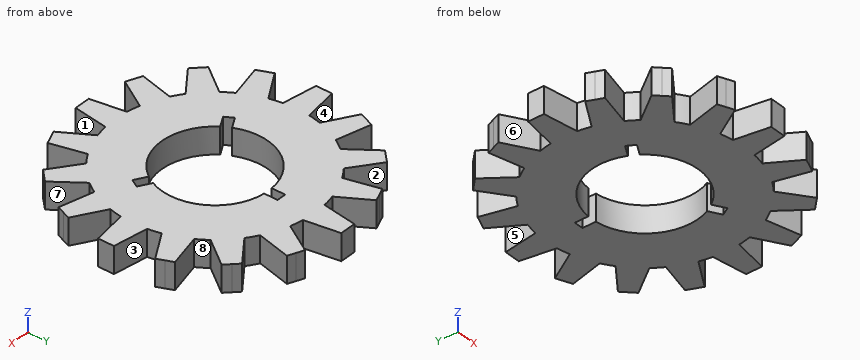
from build123d import *

# Parameters (mm, degrees)
F1_DEPTH = 2.54


with BuildPart() as f1:
    # F0 (on Top) → F1 (new body)
    with BuildSketch(Plane.XY):
        with BuildLine():
            Line((-9.5190714883, 8.4414407538), (-7.564357968, 5.788446556))
            ThreePointArc((-7.564357968, 5.788446556), (-7.9197480572, 5.2918064695), (-8.242581769, 4.7734129071))
            Line((-8.242581769, 4.7734129071), (-11.4416652874, 5.5640757948))
            Line((-11.4416652874, 5.5640757948), (-11.7332700629, 4.860079591))
            Line((-11.7332700629, 4.860079591), (-12.0248748384, 4.1560833873))
            Line((-12.0248748384, 4.1560833873), (-9.2036980994, 2.4530728273))
            ThreePointArc((-9.2036980994, 2.4530728273), (-9.3419797958, 1.8582353172), (-9.4418586268, 1.2557590022))
            Line((-9.4418586268, 1.2557590022), (-12.7, 0.762))
            Line((-12.7, 0.762), (-12.7, 0))
            Line((-12.7, 0), (-12.7, -0.762))
            Line((-12.7, -0.762), (-9.4418586268, -1.2557590022))
            ThreePointArc((-9.4418586268, -1.2557590022), (-9.3419797958, -1.8582353172), (-9.2036980994, -2.4530728273))
            Line((-9.2036980994, -2.4530728273), (-12.0248748384, -4.1560833873))
            Line((-12.0248748384, -4.1560833873), (-11.7332700629, -4.860079591))
            Line((-11.7332700629, -4.860079591), (-11.4416652874, -5.5640757948))
            Line((-11.4416652874, -5.5640757948), (-8.242581769, -4.7734129071))
            ThreePointArc((-8.242581769, -4.7734129071), (-7.9197480572, -5.2918064695), (-7.564357968, -5.788446556))
            Line((-7.564357968, -5.788446556), (-9.5190714883, -8.4414407538))
            Line((-9.5190714883, -8.4414407538), (-8.9802561211, -8.9802561211))
            Line((-8.9802561211, -8.9802561211), (-8.4414407538, -9.5190714883))
            Line((-8.4414407538, -9.5190714883), (-5.788446556, -7.564357968))
            ThreePointArc((-5.788446556, -7.564357968), (-5.2918064695, -7.9197480572), (-4.7734129071, -8.242581769))
            Line((-4.7734129071, -8.242581769), (-5.5640757948, -11.4416652874))
            Line((-5.5640757948, -11.4416652874), (-4.860079591, -11.7332700629))
            Line((-4.860079591, -11.7332700629), (-4.1560833873, -12.0248748384))
            Line((-4.1560833873, -12.0248748384), (-2.4530728273, -9.2036980994))
            ThreePointArc((-2.4530728273, -9.2036980994), (-1.8582353172, -9.3419797958), (-1.2557590022, -9.4418586268))
            Line((-1.2557590022, -9.4418586268), (-0.762, -12.7))
            Line((-0.762, -12.7), (0, -12.7))
            Line((0, -12.7), (0.762, -12.7))
            Line((0.762, -12.7), (1.2557590022, -9.4418586268))
            ThreePointArc((1.2557590022, -9.4418586268), (1.8582353172, -9.3419797958), (2.4530728273, -9.2036980994))
            Line((2.4530728273, -9.2036980994), (4.1560833873, -12.0248748384))
            Line((4.1560833873, -12.0248748384), (4.860079591, -11.7332700629))
            Line((4.860079591, -11.7332700629), (5.5640757948, -11.4416652874))
            Line((5.5640757948, -11.4416652874), (4.7734129071, -8.242581769))
            ThreePointArc((4.7734129071, -8.242581769), (5.2918064695, -7.9197480572), (5.788446556, -7.564357968))
            Line((5.788446556, -7.564357968), (8.4414407538, -9.5190714883))
            Line((8.4414407538, -9.5190714883), (8.9802561211, -8.9802561211))
            Line((8.9802561211, -8.9802561211), (9.5190714883, -8.4414407538))
            Line((9.5190714883, -8.4414407538), (7.564357968, -5.788446556))
            ThreePointArc((7.564357968, -5.788446556), (7.9197480572, -5.2918064695), (8.242581769, -4.7734129071))
            Line((8.242581769, -4.7734129071), (11.4416652874, -5.5640757948))
            Line((11.4416652874, -5.5640757948), (11.7332700629, -4.860079591))
            Line((11.7332700629, -4.860079591), (12.0248748384, -4.1560833873))
            Line((12.0248748384, -4.1560833873), (9.2036980994, -2.4530728273))
            ThreePointArc((9.2036980994, -2.4530728273), (9.3419797958, -1.8582353172), (9.4418586268, -1.2557590022))
            Line((9.4418586268, -1.2557590022), (12.7, -0.762))
            Line((12.7, -0.762), (12.7, 0))
            Line((12.7, 0), (12.7, 0.762))
            Line((12.7, 0.762), (9.4418586268, 1.2557590022))
            ThreePointArc((9.4418586268, 1.2557590022), (9.3419797958, 1.8582353172), (9.2036980994, 2.4530728273))
            Line((9.2036980994, 2.4530728273), (12.0248748384, 4.1560833873))
            Line((12.0248748384, 4.1560833873), (11.7332700629, 4.860079591))
            Line((11.7332700629, 4.860079591), (11.4416652874, 5.5640757948))
            Line((11.4416652874, 5.5640757948), (8.242581769, 4.7734129071))
            ThreePointArc((8.242581769, 4.7734129071), (7.9197480572, 5.2918064695), (7.564357968, 5.788446556))
            Line((7.564357968, 5.788446556), (9.5190714883, 8.4414407538))
            Line((9.5190714883, 8.4414407538), (8.9802561211, 8.9802561211))
            Line((8.9802561211, 8.9802561211), (8.4414407538, 9.5190714883))
            Line((8.4414407538, 9.5190714883), (5.788446556, 7.564357968))
            ThreePointArc((5.788446556, 7.564357968), (5.2918064695, 7.9197480572), (4.7734129071, 8.242581769))
            Line((4.7734129071, 8.242581769), (5.5640757948, 11.4416652874))
            Line((5.5640757948, 11.4416652874), (4.860079591, 11.7332700629))
            Line((4.860079591, 11.7332700629), (4.1560833873, 12.0248748384))
            Line((4.1560833873, 12.0248748384), (2.4530728273, 9.2036980994))
            ThreePointArc((2.4530728273, 9.2036980994), (1.8582353172, 9.3419797958), (1.2557590022, 9.4418586268))
            Line((1.2557590022, 9.4418586268), (0.762, 12.7))
            Line((0.762, 12.7), (0, 12.7))
            Line((0, 12.7), (-0.762, 12.7))
            Line((-0.762, 12.7), (-1.2557590022, 9.4418586268))
            ThreePointArc((-1.2557590022, 9.4418586268), (-1.8582353172, 9.3419797958), (-2.4530728273, 9.2036980994))
            Line((-2.4530728273, 9.2036980994), (-4.1560833873, 12.0248748384))
            Line((-4.1560833873, 12.0248748384), (-4.860079591, 11.7332700629))
            Line((-4.860079591, 11.7332700629), (-5.5640757948, 11.4416652874))
            Line((-5.5640757948, 11.4416652874), (-4.7734129071, 8.242581769))
            ThreePointArc((-4.7734129071, 8.242581769), (-5.2918064695, 7.9197480572), (-5.788446556, 7.564357968))
            Line((-5.788446556, 7.564357968), (-8.4414407538, 9.5190714883))
            Line((-8.4414407538, 9.5190714883), (-8.9802561211, 8.9802561211))
            Line((-8.9802561211, 8.9802561211), (-9.5190714883, 8.4414407538))
        make_face()
        with BuildLine():
            ThreePointArc((-4.6047852038, -2.1453095877), (-4.3994090512, 2.54), (-0.4445, 5.0605157593))
            Line((-0.4445, 5.0605157593), (-0.4445, 6.35))
            Line((-0.4445, 6.35), (0, 6.35))
            Line((0, 6.35), (0.4445, 6.35))
            Line((0.4445, 6.35), (0.4445, 5.0605157593))
            ThreePointArc((0.4445, 5.0605157593), (4.3994090512, 2.54), (4.6047852038, -2.1453095877))
            Line((4.6047852038, -2.1453095877), (5.721511314, -2.790051708))
            Line((5.721511314, -2.790051708), (5.277011314, -3.559948292))
            Line((5.277011314, -3.559948292), (4.1602852038, -2.9152061716))
            ThreePointArc((4.1602852038, -2.9152061716), (0, -5.08), (-4.1602852038, -2.9152061716))
            Line((-4.1602852038, -2.9152061716), (-5.277011314, -3.559948292))
            Line((-5.277011314, -3.559948292), (-5.721511314, -2.790051708))
            Line((-5.721511314, -2.790051708), (-4.6047852038, -2.1453095877))
        make_face(mode=Mode.SUBTRACT)
    extrude(amount=F1_DEPTH)


solid = f1.part
Can you work these out from the model? Positions are in its coordinate system, mm. Face numbers are marked on the shaded views. A direction names the side the tool comes from. Round coordinates to 2 decimals unless told otherwise and drop trailing zeros. Loops run counter-clockwise (first coordinate to the right, second up) from the corner with the lowest first, then second, coordinate; pieces in that order, holes last. Notation, with made-up numbers: (4, 40.5) - (43, 40.5) arc R15 ccw to (43, 54.5) - close; hole circle Ø7 at (-29.75, 23.5). An arc over 180 degrees is marked (long way). Write item = value, one per line. Start each with the question number.
(1) If we section it at A-A (y = -11): Please give me the cut outline in (x, z), and give its area (3 significant figures).
(2) For P1, Ø1.4, axis at y = 6, z = 2, coming from the -X side; P2, Ø10, axis at x = 2, y = 2.5, coming from the +Z side; P3, Ø1.5, axis at x = 6, z = 0.5, coming from the +Y side; P4, Ø0.6, axis at y = 5.5, z = 1, coming from the +X side, each with a flat end and sliding along its axis, tell me the tip position at first contact or that it passes through.
(3) If we section it at D-D (x = 0): Please give me the cut outline in (y, z), and give its area (3 significant figures).
(4) If we section it at B-B (x = -3): Please give me the cut outline in (y, z), and give its area (3 significant figures).
(5) If we mould it in two halves opening along X, with no side actions, what happens to the marked faces 1, 2, 3 and 4? For each: released by +X, released by -X, zero draft, split by the parting line, or undercut.
(6) For the marked faces 5, 6, 7 and 8, which set-ups out of +Z, -Z, +X, -X, +Y, -Y let a thin tool reach every point of the face, with its end or its side?
(7) If I drill on probe 1 along X at (y, z) = (-8, 0.7); probe 2 along Y at (x, z) = (11.5, 2.45); probe 3 along X at (y, z) = (-11.25, 1.95), over which ranges is the centre line in solid material (lowest first)? Write a range as [from, to].
(8) If we section it at C-C (x = 10): Please give me the cut outline in (y, z).
Ans:
q1.outline = (-5.45, 0) - (-3.54, 0) - (-3.54, 2.54) - (-5.45, 2.54) - close; (-1.02, 0) - (1.02, 0) - (1.02, 2.54) - (-1.02, 2.54) - close; (3.54, 0) - (5.45, 0) - (5.45, 2.54) - (3.54, 2.54) - close
q1.area = 14.9 mm²
q2.P1 = -11.55
q2.P2 = 2.54
q2.P3 = 11.57
q2.P4 = 11.59
q3.outline = (-12.7, 0) - (-5.08, 0) - (-5.08, 2.54) - (-12.7, 2.54) - close; (6.35, 0) - (12.7, 0) - (12.7, 2.54) - (6.35, 2.54) - close
q3.area = 35.5 mm²
q4.outline = (-10.11, 0) - (-4.1, 0) - (-4.1, 2.54) - (-10.11, 2.54) - close; (4.1, 0) - (10.11, 0) - (10.11, 2.54) - (4.1, 2.54) - close
q4.area = 30.5 mm²
q5.face_1 = undercut
q5.face_2 = undercut
q5.face_3 = released by +X
q5.face_4 = released by -X
q6.face_5 = +Z, -Z, +Y
q6.face_6 = +Z, -Z, -X
q6.face_7 = +Z, -Z, +X
q6.face_8 = +Z, -Z
q7.probe_1 = [-9.19, -6.38], [-5.17, 5.17], [6.38, 9.19]
q7.probe_2 = [-5.42, -3.84], [-0.94, 0.94], [3.84, 5.42]
q7.probe_3 = [-5.52, -3.69], [-0.98, 0.98], [3.69, 5.52]
q8.outline = (-5.21, 0) - (-2.93, 0) - (-2.93, 2.54) - (-5.21, 2.54) - close; (-1.17, 0) - (1.17, 0) - (1.17, 2.54) - (-1.17, 2.54) - close; (2.93, 0) - (5.21, 0) - (5.21, 2.54) - (2.93, 2.54) - close
